CAD build for the part. Positions are in the model's coordinates, mm. A direction names the side the tool comes from. Coordinates: 2 decimals unless noted, no trailing zeros. Loops run counter-clockwise (first coordinate to the right, second up) from the corner with the lowest first, then second, coordinate; pieces in that order, holes last. Notation, with made-up numbers: (-5, 3) -> (5, 3) arc R15 cw to (5, 28) -> close; hole circle Ø11 at (-22.5, 7). An arc over 180 degrees is marked (long way). Write each question's results on one line, items separated by ' | '.
from build123d import *

# Parameters (mm, degrees)
F0_W     = 63.703202
F0_H     = 49.072805
F0_R     = 9.207281
F1_DEPTH = 30.988
F2_W     = 46.3296
F2_H     = 48.767999
F2_R     = 8.252146
F3_DEPTH = 8.89
F4_W     = 110.642403
F4_H     = 68.580005
F5_DEPTH = 10.668


with BuildPart() as f1:
    # F0 (on Top) → F1 (new body)
    with BuildSketch(Plane.XY):
        with Locations((-34.594801, 11.277599)):
            Rectangle(F0_W, F0_H)
        with Locations((-34.594801, 11.2776)):
            Circle(F0_R, mode=Mode.SUBTRACT)
    extrude(amount=F1_DEPTH)

    # F2 (on Top) → F3 (join)
    with BuildSketch(Plane.XY):
        with Locations((20.1168, 11.125199)):
            Rectangle(F2_W, F2_H)
        with Locations((20.1168, 11.125199)):
            Circle(F2_R, mode=Mode.SUBTRACT)
    extrude(amount=F3_DEPTH)

    # F4 (on face) → F5 (join)
    with BuildSketch(Plane(origin=(0, 0, 0), x_dir=(1, 0, 0), z_dir=(0, 0, -1))):
        with Locations((-11.734799, -12.192001)):
            Rectangle(F4_W, F4_H)
    extrude(amount=F5_DEPTH)


solid = f1.part
1) Pin check, flat tips, straight feed: pin 1 (8 mm diameter, centred on y = 13.5, z = 20.5, fed in from -X); pin 2 (13 mm diameter, centred on x = 20.12, y = 11.13, fed in from +Z); pin 3 (7 mm diameter, centred on x = 13, z = 6, fed in from -Y); pin 4 (8 mm diameter, centred on x = -35.5, z = 2, fed in from -Y). Stop position of each tip, or through.
Outcome:
pin 1: stops at x = -66.45 | pin 2: stops at z = 0 | pin 3: stops at y = -13.26 | pin 4: stops at y = -22.1
2) Slice it at B-B (x = -47.5). Write the cut outline in (y, z), then the cut area to 3 significant figures.
Outcome:
outline: (-22.1, -10.67) -> (46.48, -10.67) -> (46.48, 0) -> (35.81, 0) -> (35.81, 30.99) -> (-13.26, 30.99) -> (-13.26, 0) -> (-22.1, 0) -> close | area: 2,250 mm^2
3) Slice it at C-C (z = 13.5). Write the cut outline in (x, y).
Outcome:
outline: (-66.45, -13.26) -> (-2.74, -13.26) -> (-2.74, 35.81) -> (-66.45, 35.81) -> close; hole circle Ø18.41 at (-34.59, 11.28)
4) Slice it at A-A (y = 27.5). Write the cut outline in (x, z), then the cut area to 3 significant figures.
Outcome:
outline: (-67.06, -10.67) -> (43.59, -10.67) -> (43.59, 0) -> (43.28, 0) -> (43.28, 8.89) -> (-2.74, 8.89) -> (-2.74, 30.99) -> (-66.45, 30.99) -> (-66.45, 0) -> (-67.06, 0) -> close | area: 3,560 mm^2
5) Drill centre lines: L1, parallel to Y at x = -22, z = 16; L2, parallel to Z at x = 14, y = -13; L3, parallel to Y at x = -28, z = 18. Where is each one in solid material? Low to high. Write a range as from..to.
Outcome:
L1: y = -13.26..35.81 | L2: z = -10.67..8.89 | L3: y = -13.26..4.85, 17.7..35.81
6) Slice it at D-D (x = 2). Write the cut outline in (y, z).
Outcome:
outline: (-22.1, -10.67) -> (46.48, -10.67) -> (46.48, 0) -> (35.51, 0) -> (35.51, 8.89) -> (-13.26, 8.89) -> (-13.26, 0) -> (-22.1, 0) -> close
7) Which spindle directions (+Z, -Z, +X, -X, +Y, -Y) get a long thin tool onto all of the face, cutting with end or side? Do faces 5 (the cylindrical face through (13.57, 6.1, 4.38)), 6 (the flat face through (-35, 35.814, 15)), 7 (the flat face through (-66.446, 11, 15)). Say none if no direction does.
Outcome:
face 5: +Z | face 6: +Z, +X, -X, +Y | face 7: +Z, -X, +Y, -Y
8) Two-plate mould, pull along X, no slides. Class faces 1 (the cylindrical face through (-41.38, 17.5, 15.28)), 2 (the flat face through (10, 11, 8.89)), 3 (the flat face through (43.282, 11, 4)), 4 (the flat face through (20, 11, 0)): pulls with the +X half, pulls with the -X half, needs draft (parallel to the pull), parting line crosses it, or undercut.
Outcome:
face 1: undercut | face 2: needs draft | face 3: pulls with the +X half | face 4: undercut
